Can you work these out from the model? Positions are in its coordinate system, mm. A direction names the side the tool comes from. Give positions to 0.01 mm unless a question says otherwise; leave off trailing zeros. Loops run counter-clockwise (first coordinate to the right, second up) from the corner with the lowest first, then second, coordinate; pieces in that order, holes last. Notation, with made-up numbers: (5, -20) - (54, -20) arc R22 cw to (54, 15) - close; hole circle Ø11 at (21, 62.5). An arc over 180 degrees is marked (long way). Answer as a JSON object with one key per item and string values.
```python
from build123d import *

# Parameters (mm, degrees)
F0_W     = 58.9387752116
F0_H     = 49.3731051683
F1_DEPTH = 134.7465757281
F2_R     = 16.9673265676
F3_DEPTH = 58.9397752116
F4_R     = 12.7
F7_DEPTH = 203.2
F9_DEPTH = 203.201


with BuildPart() as f1:
    # F0 (on Top) → F1 (new body)
    with BuildSketch(Plane.XY):
        with Locations((3.1067002565, 0.1738145947)):
            Rectangle(F0_W, F0_H)
    extrude(amount=F1_DEPTH)

    # F2 (on face) → F3 (cut, through all)
    with BuildSketch(Plane(origin=(-26.3626873493, 0, 0), x_dir=(0, -1, 0), z_dir=(-1, 0, 0))):
        with Locations((10.2675408125, 109.3456819654)):
            Circle(F2_R)
    extrude(amount=-F3_DEPTH, mode=Mode.SUBTRACT)

    # F4
    f4_edges = [f1.edges().sort_by_distance(p)[0] for p in [
        (32.576088, 0.173815, 134.746576),
    ]]
    fillet(f4_edges, radius=F4_R)


with BuildPart() as f7:
    # F6 (on Right) → F7 (new body)
    with BuildSketch(Plane.YZ):
        Polygon((33.2775712013, 15.3340250254), (33.2775712013, 43.1480407715), (-43.289065361, 15.3340250254), align=None)
    extrude(amount=F7_DEPTH)

    # F8 (on face) → F9 (cut, through all)
    with BuildSketch(Plane.YZ.offset(203.2)):
        Polygon((26.9275712013, 34.0853054408), (-24.6910978089, 15.3340250254), (26.9275712013, 15.3340250254), align=None)
    extrude(amount=-F9_DEPTH, mode=Mode.SUBTRACT)


solid = f7.part
```
1) Imagine slicing it at A-A on z = 19.25. Write out the boundary of the cut face in (x, y), and give its area (3 significant figures).
Check sheet entries:
{"outline": "(0, -32.51) - (203.2, -32.51) - (203.2, -13.91) - (0, -13.91) - close; (0, 26.93) - (203.2, 26.93) - (203.2, 33.28) - (0, 33.28) - close", "area": "5,070 mm2"}
2) Imagine slicing it at D-D on z = 39. Write out the boundary of the cut face in (x, y), and give its area (3 significant figures).
Check sheet entries:
{"outline": "(0, 21.86) - (203.2, 21.86) - (203.2, 33.28) - (0, 33.28) - close", "area": "2,320 mm2"}
3) I'm going to push a flat-ended pin straight in: P1, Ø10, axis at y = -27, z = 30.5, coming from the -X side. Where does the tip first touch, or does it pass through?
Check sheet entries:
{"P1": "through"}
4) Imagine slicing it at C-C on y = -28.5. Write out the boundary of the cut face in (x, z), and give its area (3 significant figures).
Check sheet entries:
{"outline": "(0, 15.33) - (203.2, 15.33) - (203.2, 20.71) - (0, 20.71) - close", "area": "1,090 mm2"}
5) Imagine slicing it at B-B on x = 53.5. Write out the boundary of the cut face in (y, z), and give its area (3 significant figures).
Check sheet entries:
{"outline": "(-43.29, 15.33) - (-24.69, 15.33) - (26.93, 34.09) - (26.93, 15.33) - (33.28, 15.33) - (33.28, 43.15) - close", "area": "581 mm2"}
6) Which directions (+Z, -Z, +X, -X, +Y, -Y) give clear straight access to the entire face, cutting with the end or side of a thin tool? Please do faces 1 (the flat face through (103, 26.928, 25)), 2 (the flat face through (100, 33.278, 29)).
Check sheet entries:
{"face 1": "-Z, +X, -X", "face 2": "+Z, -Z, +X, -X, +Y"}
7) I need wall thicknesses on L1, parallel to Z at x = 18, y = 20.5; L2, parallel to Z at x = 150.5, y = -24.5. Which ranges of each line are inside material? Lowest first, please.
Check sheet entries:
{"L1": "31.75 to 38.51", "L2": "15.4 to 22.16"}
